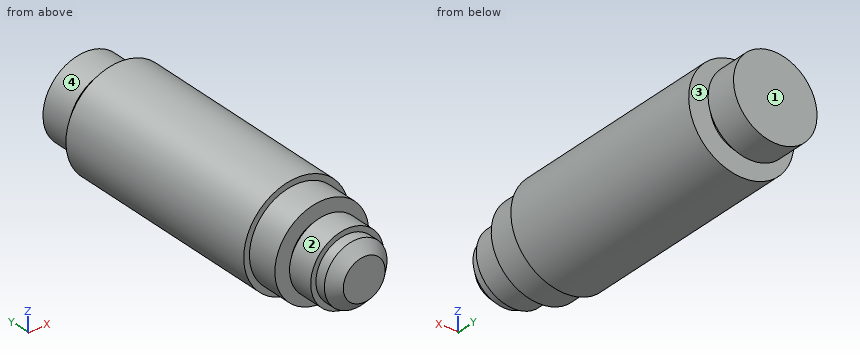
```python
from build123d import *

# Parameters (mm, degrees)
CHAMFER1_SIZE = 2.54


with BuildPart() as part:
    # Sketch1 → Revolve1 (revolve)
    with BuildSketch(Plane.XY, mode=Mode.PRIVATE) as revolve1_sk:
        Polygon((12.827, 73.66), (12.827, 20.32), (11.43, 20.32), (11.43, 12.7), (7.62, 12.7), (7.62, 11.43), (8.89, 11.43), (8.89, 5.08), (7.62, 5.08), (7.62, 2.54), (5.08, 2.54), (5.08, 0), (0, 0), (0, 83.82), (10.16, 83.82), (10.16, 76.2), (7.62, 76.2), (7.62, 73.66), align=None)
    revolve(revolve1_sk.sketch.rotate(Axis((0, 0, 0), (0, 1, 0)), 90), axis=Axis((0, 0, 0), (0, 1, 0)))

    # Chamfer1
    chamfer1_edges = [part.edges().sort_by_distance(p)[0] for p in [
        (0, 2.54, 5.08),
    ]]
    chamfer(chamfer1_edges, length=CHAMFER1_SIZE - 0.0001)  # a hair under: the kernel refuses the full size


solid = part.part
```
CAD build for the part. Positions are in the model's coordinates, mm. Face numbers are marked on the shaded views. A direction names the side the tool comes from. Coordinates: 2 decimals unless noted, no trailing zeros. Loops run counter-clockwise (first coordinate to the right, second up) from the corner with the lowest first, then second, coordinate; pieces in that order, holes last. Notation, with made-up numbers: (-19, 15) - (-11, 15) arc R9 ccw to (-11, 24) - close; hole circle Ø5 at (39.5, -32.75). An arc over 180 degrees is marked (long way). Return JSON: item names as keys, results as strings.
1. Band-saw the part on D-D (y = 24.5). Give the cut face in (x, z), and give its area (3 significant figures).
Result:
{"outline": "circle Ø25.65 at (0, 0)", "area": "517 mm2"}
2. Probe L1, parallel to Y at x = 8.5, z = 1; L2, parallel to Z at x = 0.25, y = 31.5; L3, parallel to X at y = 15, z = -0.25. List the from-to ranges inside material, lowest first. Write a range as from..to.
Result:
{"L1": "y = 5.08..11.43, 12.7..73.66, 76.2..83.82", "L2": "z = -12.82..12.82", "L3": "x = -11.43..11.43"}
3. Drop flat-ended pins along their axis: pin 1 (12 mm diameter, centred on x = -7, y = 40, fed in from +Z); pin 2 (1 mm diameter, centred on y = 16.5, z = -5.5, fed in from -X); pin 3 (8 mm diameter, centred on x = -1, z = 5.5, fed in from -Y); pin 4 (3 mm diameter, centred on x = -4, y = 26.5, fed in from -Z). Give the stop position or say it passes through.
Result:
{"pin 1": "stops at z = 12.79", "pin 2": "stops at x = -10.28", "pin 3": "stops at y = 0", "pin 4": "stops at z = -12.58"}
4. 3-axis set-ups, long thin cutter, end or side, ignore diameter. For the marked faces 1, 2, 3 and 4: which of +Z, -Z, +X, -X, +Y, -Y reach the whole face in a straight line?
Result:
{"face 1": "+Z, -Z, +X, -X, +Y", "face 2": "-Y", "face 3": "none", "face 4": "+Y"}
5. Band-saw the part on C-C (y = 8). Give the cut face in (x, z).
Result:
{"outline": "circle Ø17.78 at (0, 0)"}
